Verification items for the finished model (mm, model axes). A direction names the side the tool comes from. Give positions to 0.01 mm unless a question says otherwise; leave off trailing zeros. Loops run counter-clockwise (first coordinate to the right, second up) from the corner with the lowest first, then second, coordinate; pieces in that order, holes last. Notation, with made-up numbers: (64, 50) - (71, 50) arc R19 ccw to (71, 80) - close; hole circle Ø1 at (-28.75, 36.25). An arc over 180 degrees is marked (long way). Answer in a Markdown table with one row per item.
```python
from build123d import *

# Parameters (mm, degrees)
SKETCH1_R           = 1.7018
SKETCH1_R_2         = 1.1
BOSS_EXTRUDE1_DEPTH = 3.175


with BuildPart() as part:
    # Sketch1 → Boss-Extrude1 (new body)
    with BuildSketch(Plane.XY):
        with BuildLine():
            Line((-23.059785094, 18.235838692), (-8.221884337, 0))
            Line((-8.221884337, 0), (-23.059785094, -18.235838692))
            ThreePointArc((-23.059785094, -18.235838692), (-23.396423143, -18.732811969), (-23.641240585, -19.280874041))
            Line((-23.641240585, -19.280874041), (-26.436877512, -27.377570282))
            ThreePointArc((-26.436877512, -27.377570282), (-24.163274934, -33.322252318), (-17.913202642, -32.120125223))
            Line((-17.913202642, -32.120125223), (0, -10.104728355))
            Line((0, -10.104728355), (17.913202642, -32.120125223))
            ThreePointArc((17.913202642, -32.120125223), (24.163274934, -33.322252318), (26.436877512, -27.377570282))
            Line((26.436877512, -27.377570282), (23.641240585, -19.280874041))
            ThreePointArc((23.641240585, -19.280874041), (23.396423143, -18.732811969), (23.059785094, -18.235838692))
            Line((23.059785094, -18.235838692), (8.221884337, 0))
            Line((8.221884337, 0), (23.059785094, 18.235838692))
            ThreePointArc((23.059785094, 18.235838692), (23.396423143, 18.732811969), (23.641240585, 19.280874041))
            Line((23.641240585, 19.280874041), (26.436877512, 27.377570282))
            ThreePointArc((26.436877512, 27.377570282), (24.163274934, 33.322252318), (17.913202642, 32.120125223))
            Line((17.913202642, 32.120125223), (0, 10.104728355))
            Line((0, 10.104728355), (-17.913202642, 32.120125223))
            ThreePointArc((-17.913202642, 32.120125223), (-24.163274934, 33.322252318), (-26.436877512, 27.377570282))
            Line((-26.436877512, 27.377570282), (-23.641240585, 19.280874041))
            ThreePointArc((-23.641240585, 19.280874041), (-23.396423143, 18.732811969), (-23.059785094, 18.235838692))
        make_face()
        with Locations((21.7551, 28.9941)):
            Circle(SKETCH1_R, mode=Mode.SUBTRACT)
        with Locations((-21.7551, 28.9941)):
            Circle(SKETCH1_R, mode=Mode.SUBTRACT)
        with Locations((-21.7551, -28.9941)):
            Circle(SKETCH1_R, mode=Mode.SUBTRACT)
        with Locations((21.7551, -28.9941)):
            Circle(SKETCH1_R, mode=Mode.SUBTRACT)
        with Locations((20.40001, 20.40001)):
            Circle(SKETCH1_R_2, mode=Mode.SUBTRACT)
        with Locations((-20.40001, 20.40001)):
            Circle(SKETCH1_R_2, mode=Mode.SUBTRACT)
        with Locations((-20.40001, -20.40001)):
            Circle(SKETCH1_R_2, mode=Mode.SUBTRACT)
        with Locations((20.40001, -20.40001)):
            Circle(SKETCH1_R_2, mode=Mode.SUBTRACT)
    extrude(amount=BOSS_EXTRUDE1_DEPTH)


solid = part.part
```
Q1. Tool access check on faces 4 (the face through (-9.082, -21.267, 1.565)), 5 (the face through (-25.06, 23.39, 1.57)), 6 (the face through (-8.83, 20.96, 1.57)), 7 (the face through (15.537, 8.99, 1.565)), 8 (the face through (21.416, -20.821, 1.565)). Record the directions out of +Z, -Z, +X, -X, +Y, -Y that give a thin tool (end or side, any length) a straight path to the whole face; none if there is none.
Completed:
| item | result |
|---|---|
| face 4 | +Z, -Z, -Y |
| face 5 | +Z, -Z, -X |
| face 6 | +Z, -Z, +Y |
| face 7 | +Z, -Z, +X |
| face 8 | +Z, -Z |
Q2. Go/stop test with flat-tipped pins: P1, Ø3, axis at x = -20.4, y = -20.4, coming from the +Z side (3 decimals); P2, Ø1.5, axis at x = 10.5, z = 1.5, coming from the +Y side; P3, Ø1.5, axis at y = -6.5, z = 0.5, coming from the -X side; P4, Ø1.5, axis at x = 20.5, z = 2.5, coming from the +Y side. Record where each tip stops, or that it passes through.
Completed:
| item | result |
|---|---|
| P1 | z = 3.175 |
| P2 | y = 23.93 |
| P3 | x = -14.12 |
| P4 | y = 33.92 |
Q3. Sectioned sample at A-A (x = -10.5). Record the cut outline in (y, z) (3 decimals), and give its area (3 significant figures).
Completed:
| item | result |
|---|---|
| outline | (-23.009, 0) - (-2.8, 0) - (-2.8, 3.175) - (-23.009, 3.175) - close; (2.8, 0) - (23.009, 0) - (23.009, 3.175) - (2.8, 3.175) - close |
| area | 128 mm^2 |
Q4. Sectioned sample at C-C (z = 2.55). Give the number of separate pieces and of enclosed holes in the cut face, and give its area (3 significant figures).
Completed:
| item | result |
|---|---|
| separate pieces | 1 |
| enclosed holes | 8 |
| area | 1,750 mm^2 |
Q5. Sectioned sample at D-D (x = 2). Record the cut outline in (y, z) (3 decimals), and give its area (3 significant figures).
Completed:
| item | result |
|---|---|
| outline | (-12.563, 0) - (12.563, 0) - (12.563, 3.175) - (-12.563, 3.175) - close |
| area | 79.8 mm^2 |
Q6. Thickness scan on line 1 (Y direction, x = 20.5, z = 2.1); line 2 (X direction, y = 0, z = 2.2); line 3 (X direction, y = 26, z = 0.35). Record the ranges inside material, lowest first.
Completed:
| item | result |
|---|---|
| line 1 | -33.79 to -30.14, -27.84 to -21.5, -19.3 to -15.09, 15.09 to 19.3, 21.5 to 27.84, 30.14 to 33.79 |
| line 2 | -8.22 to 8.22 |
| line 3 | -25.96 to -12.93, 12.93 to 25.96 |
Q7. Draft check along X on faces 1 (the face through (-25.02, -23.27, 1.57)), 2 (the face through (25.02, 23.27, 1.57)), 3 (the face through (8.83, -20.96, 1.57)). Enter one of: +X half, -X half, draft (parallel to the pull), parting line (faces both ways), or undercut.
Completed:
| item | result |
|---|---|
| face 1 | -X half |
| face 2 | +X half |
| face 3 | undercut |
Q8. Sectioned sample at B-B (y = -12). Record the cut outline in (x, z) (3 decimals), and give its area (3 significant figures).
Completed:
| item | result |
|---|---|
| outline | (-17.986, 0) - (-1.542, 0) - (-1.542, 3.175) - (-17.986, 3.175) - close; (1.542, 0) - (17.986, 0) - (17.986, 3.175) - (1.542, 3.175) - close |
| area | 104 mm^2 |
